from build123d import *

# Parameters (mm, degrees)
F3_W     = 8
F3_H     = 1
F4_DEPTH = 2.4


with BuildPart() as f1:
    # F0 (on Front) → F1 (revolve)
    with BuildSketch(Plane.XZ):
        with BuildLine():
            Line((0, 17.697224), (0, 0))
            Line((0, 0), (1.1, 1.1))
            Line((1.1, 1.1), (1.5, 13))
            Line((1.5, 13), (3, 16))
            ThreePointArc((3, 16), (1.72341, 17.24351), (0, 17.697224))
        make_face()
    revolve(axis=Axis((0, 0, 8.848612), (0, 0, 1)))

    # F3 (on offset) → F4 (cut)
    with BuildSketch(Plane.XY.offset(16)):
        Rectangle(F3_W, F3_H)
    extrude(amount=F4_DEPTH, mode=Mode.SUBTRACT)


solid = f1.part
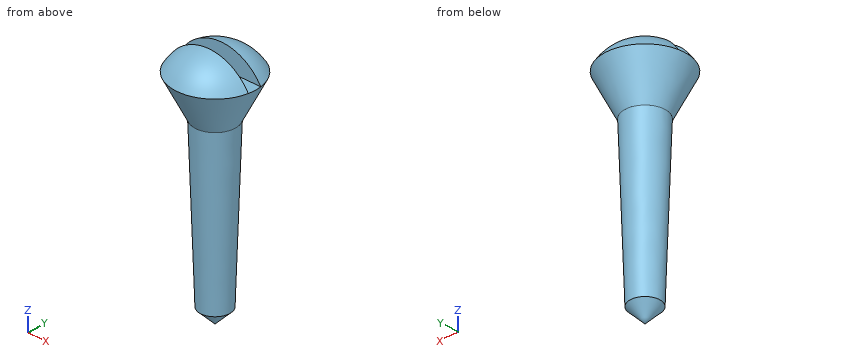
For this review, take the finished solid that the model builds, in its own axes (mm). Round coordinates to 2 decimals unless told otherwise and drop trailing zeros. Write each loop counter-clockwise with the first axis right and the second up, starting at its lowest first coordinate (ties: lowest second). Pieces come first, ordered by that corner, then holes. Notation, with made-up numbers: (41, -39) - (47, -39) arc R16 ccw to (47, -9) - close; hole circle Ø3 at (70.25, -26.5). An arc over 180 degrees is marked (long way). Write item = value, one per line. Start each with the question number.
1. Wall thickness on L1, parallel to X at y = -1, z = 9.25; L2, parallel to Z at x = 2.5, y = -1; L3, parallel to Y at x = 0, z = 8.25: over which ranges is each line inside the solid? List them lowest first.
2. For pin 1 Ø1 at (x, y) = (2, 0.5) entering from +Z; pin 2 Ø0.8 at (x, z) = (-1.5, 16.5) entering from -Y; pin 3 Ø0.8 at (x, z) = (-0.5, 17) entering from +Y, all flat-tipped, find the tip position at first contact; note any pin that passes through.
3. Consider section A-A on z = 15.5. State the section outline as (x, y) points.
4. Consider section B-B on z = 3.75. State the section outline as (x, y) points, plus the area to 3 significant figures.
Evaluation:
q1.L1 = -0.94 to 0.94
q1.L2 = 15.39 to 16.43
q1.L3 = -1.34 to 1.34
q2.pin_1 = 17.32
q2.pin_2 = -2.6
q2.pin_3 = 2.5
q3.outline = circle Ø5.5 at (0, 0)
q4.outline = circle Ø2.38 at (0, 0)
q4.area = 4.44 mm2
